```python
from build123d import *

# Parameters (mm, degrees)
SKETCH001_R       = 0.65
PAD001_DEPTH      = 10.5
PAD001_DEPTH_BACK = 3.5
SKETCH_R          = 6
PAD_DEPTH         = 21
FILLET_R          = 0.5


with BuildPart() as pad001:
    # Sketch001 → Pad001 (new body, two sides)
    with BuildSketch(Plane.XY.offset(0.5)) as pad001_sk:
        Circle(SKETCH001_R)
        with Locations((6, 0)):
            Circle(SKETCH001_R)
    extrude(amount=PAD001_DEPTH)
    extrude(pad001_sk.sketch, amount=-PAD001_DEPTH_BACK)


with BuildPart() as obj1:
    # Sketch → Pad (new body)
    with BuildSketch(Plane.XY.offset(0.1)):
        with Locations((3, 0)):
            Circle(SKETCH_R)
    extrude(amount=PAD_DEPTH)

    # Fillet
    fillet_edges = [obj1.edges().sort_by_distance(p)[0] for p in [
        (-3, 0, 0.1),
        (-3, 0, 21.1),
    ]]
    fillet(fillet_edges, radius=FILLET_R)

    add(pad001.part)


solid = obj1.part
```
Here's how the part is built. I have some questions about the finished solid (model axes, mm). Coordinates: 2 decimals unless noted, no trailing zeros. Order: outer loops, then holes, each group sorted by start corner. A loop starts at its lowest first (then second) coordinate and runs counter-clockwise, first axis right, second up. Notation, with made-up numbers: M 15.5,86.5 L 31.5,86.5 A36 cw 31.5,121.5 Z; hole C 35.25,-33 d8. An arc over 180 degrees is marked long. Answer as a JSON object with one key per item and string values. Group by question number.
(1) Suppose I cut it at A-A, the plane y = 0. Please give me the cut outline in (x, z).
(2) If we mould it in two halves opening along X, with no side actions, what happens to faces 1 (the face through (-0.085, 0.644, -1.428)), 2 (the face through (0, 0, -3)), 3 (the face through (6.62, 0.2, -1.43)), 4 (the face through (8.54, -2.3, 10.46))? For each: released by +X, released by -X, zero draft, split by the parting line, or undercut.
(3) For pin 1 (1.5 mm diameter, centred on y = -3.5, z = 14, fed in from -X); pin 2 (4 mm diameter, centred on x = 4.5, z = 12.5, fed in from +Y); pin 3 (1 mm diameter, centred on y = 1.5, z = 18.5, fed in from +X); pin 4 (2 mm diameter, centred on x = 1, y = 2.5, fed in from -Z), each with a flat end and sliding along its axis, tell me the tip position at first contact or that it passes through.
(4) Suppose I cut it at C-C, the plane z = 5.25. Please give me the cut outline in (x, y).
(5) Suppose I cut it at B-B, the plane x = 3. Please give me the cut outline in (y, z).
(6) I need wall thicknesses on probe 1 along Z at (x, y) = (6.5, 4.25); probe 2 along X at (y, z) = (-0.25, 13); probe 3 along X at (y, z) = (-4, 0.75). Which ranges of each line are inside material? Lowest first, please.
Values found:
{
 "1": {"outline": "M -3,0.6 A0.5 ccw -2.5,0.1 L -0.65,0.1 L -0.65,-3 L 0.65,-3 L 0.65,0.1 L 5.35,0.1 L 5.35,-3 L 6.65,-3 L 6.65,0.1 L 8.5,0.1 A0.5 ccw 9,0.6 L 9,20.6 A0.5 ccw 8.5,21.1 L -2.5,21.1 A0.5 ccw -3,20.6 Z"},
 "2": {"face 1": "undercut", "face 2": "zero draft", "face 3": "undercut", "face 4": "split by the parting line"},
 "3": {"pin 1": "stops at x = -2.33", "pin 2": "stops at y = 6", "pin 3": "stops at x = 8.92", "pin 4": "stops at z = 0.1"},
 "4": {"outline": "C 3,0 d12"},
 "5": {"outline": "M -6,0.6 A0.5 ccw -5.5,0.1 L 5.5,0.1 A0.5 ccw 6,0.6 L 6,20.6 A0.5 ccw 5.5,21.1 L -5.5,21.1 A0.5 ccw -6,20.6 Z"},
 "6": {"probe 1": "z = 0.1 to 21.1", "probe 2": "x = -2.99 to 8.99", "probe 3": "x = -1.47 to 7.47"}
}
